Read the model definition and answer for the solid it produces. Units are mm, in the model's axes. A direction names the side the tool comes from. Round coordinates to 2 decimals unless told otherwise and drop trailing zeros. Write each loop counter-clockwise with the first axis right and the second up, starting at its lowest first coordinate (ties: lowest second). Pieces come first, ordered by that corner, then holes.
from build123d import *

# Parameters (mm, degrees)
F0_W     = 38.1
F0_H     = 25.4
F1_DEPTH = 1.5875
F3_DEPTH = 1.5875
F5_DEPTH = 1.5885
F6_R     = 3.175
F7_DEPTH = 1.5885
F8_R     = 1.905
F9_DEPTH = 25.4


with BuildPart() as f1:
    # F0 (on Front) → F1 (new body)
    with BuildSketch(Plane.XZ):
        with Locations((19.05, 12.7)):
            Rectangle(F0_W, F0_H)
    extrude(amount=F1_DEPTH)

    # F2 (on Front) → F3 (join, through all)
    with BuildSketch(Plane.XZ):
        Polygon((43.18, 25.4), (38.1, 25.4), (38.1, 22.86), (40.64, 22.86), (40.64, 0), (43.18, -5.08), align=None)
        Polygon((-2.54, 22.86), (0, 22.86), (0, 25.4), (-5.08, 25.4), (-5.08, -5.08), (-2.54, 0), align=None)
    extrude(amount=F3_DEPTH)

    # F4 (on Front) → F5 (cut, through all)
    with BuildSketch(Plane.XZ):
        Polygon((7.62, 25.4), (2.54, 25.4), (4.2926, 20.32), (4.2926, 12.7), (5.8674, 12.7), (5.8674, 20.32), align=None)
    extrude(amount=F5_DEPTH, mode=Mode.SUBTRACT)

    # F6 (on Front) → F7 (cut, through all)
    with BuildSketch(Plane.XZ):
        with Locations((16.146441, 17.598042)):
            Circle(F6_R)
        with Locations((27.820959, 17.598042)):
            Circle(F6_R)
        with Locations((16.146441, 7.801958)):
            Circle(F6_R)
        with Locations((27.820959, 7.801958)):
            Circle(F6_R)
    extrude(amount=F7_DEPTH, mode=Mode.SUBTRACT)

    # F8 (on face) → F9 (cut)
    with BuildSketch(Plane.XZ.offset(1.5875)):
        with Locations((10.16, 0)):
            Circle(F8_R)
        with Locations((17.78, 0)):
            Circle(F8_R)
        with Locations((25.4, 0)):
            Circle(F8_R)
        with Locations((33.02, 0)):
            Circle(F8_R)
    extrude(amount=-F9_DEPTH, mode=Mode.SUBTRACT)


solid = f1.part
Q1. Section C-C (z = 3.5) is taken. Determine the outline of the cut face in (x, y), then the cut area to 3 significant figures.
Verdict:
outline: (-5.08, -1.59) - (-2.54, -1.59) - (-2.54, 0) - (-5.08, 0) - close; (0, -1.59) - (38.1, -1.59) - (38.1, 0) - (0, 0) - close; (40.64, -1.59) - (43.18, -1.59) - (43.18, 0) - (40.64, 0) - close
area: 68.5 mm2
Q2. Section B-B (x = 17.78) is taken. Determine the outline of the cut face in (y, z) (1 decimal).
Verdict:
outline: (-1.6, 1.9) - (0, 1.9) - (0, 5.1) - (-1.6, 5.1) - close; (-1.6, 10.5) - (0, 10.5) - (0, 14.9) - (-1.6, 14.9) - close; (-1.6, 20.3) - (0, 20.3) - (0, 25.4) - (-1.6, 25.4) - close
Q3. Straight lines are drawn through the part: probe 1 along X at (y, z) = (-1.05, 12.5); probe 2 along X at (y, z) = (-1.45, 14); probe 3 along X at (y, z) = (-0.75, 16). For each, find the intervals that lie inside material, in ascending order.
Verdict:
probe 1: x = -5.08 to -2.54, 0 to 38.1, 40.64 to 43.18
probe 2: x = -5.08 to -2.54, 0 to 4.29, 5.87 to 38.1, 40.64 to 43.18
probe 3: x = -5.08 to -2.54, 0 to 4.29, 5.87 to 13.4, 18.89 to 25.08, 30.56 to 38.1, 40.64 to 43.18
Q4. Flat-ended cylindrical pins translate along their axes: pin 1 Ø0.8 at (x, y) = (-2, -1) entering from -Z; pin 2 Ø0.8 at (x, y) = (37, -1) entering from -Z; pin 3 Ø7.5 at (x, z) = (27.82, 17.6) entering from -Y. Find the tip coordinate at first contact, or state that the pin passes through.
Verdict:
pin 1: stops at z = 22.86
pin 2: stops at z = 0
pin 3: stops at y = -1.59
Q5. Determine the mould class of faces 1 (the flat face through (26, -1, 25.4)), 2 (the flat face through (43.18, -1, 10)), 3 (the flat face through (5, -1, 12.7)) for opening direction X: pulls with the +X half, pulls with the -X half, needs draft (parallel to the pull), parting line crosses it, or undercut.
Verdict:
face 1: needs draft
face 2: pulls with the +X half
face 3: undercut
Q6. Which of the six approach directions +Z, -Z, +X, -X, +Y, -Y give full straight-line access (tool end or side, diameter ignored) to faces 4 (the cylindrical face through (19.08, -0.78, 16.38)), 5 (the flat face through (6.73, -0.78, 22.82)), 6 (the flat face through (4, -1, 0))?
Verdict:
face 4: +Y, -Y
face 5: +Z, +Y, -Y
face 6: -Z, +Y, -Y
Q7. Section D-D (z = 15) is taken. Determine the outline of the cut face in (x, y), then the cut area to 3 significant figures.
Verdict:
outline: (-5.08, -1.59) - (-2.54, -1.59) - (-2.54, 0) - (-5.08, 0) - close; (0, -1.59) - (4.29, -1.59) - (4.29, 0) - (0, 0) - close; (5.87, -1.59) - (14.32, -1.59) - (14.32, 0) - (5.87, 0) - close; (17.97, -1.59) - (26, -1.59) - (26, 0) - (17.97, 0) - close; (29.65, -1.59) - (38.1, -1.59) - (38.1, 0) - (29.65, 0) - close; (40.64, -1.59) - (43.18, -1.59) - (43.18, 0) - (40.64, 0) - close
area: 54.5 mm2
Q8. Section A-A (z = -0.5) is taken. Determine the outline of the cut face in (x, y).
Verdict:
outline: (-5.08, -1.59) - (-2.79, -1.59) - (-2.79, 0) - (-5.08, 0) - close; (40.89, -1.59) - (43.18, -1.59) - (43.18, 0) - (40.89, 0) - close
